Geometry check sheet. Reference: the model listing, model coordinates, mm. Round coordinates to 2 decimals unless told otherwise and drop trailing zeros. Loops run counter-clockwise (first coordinate to the right, second up) from the corner with the lowest first, then second, coordinate; pieces in that order, holes last.
```python
from build123d import *

# Parameters (mm, degrees)
F1_DEPTH = 127


with BuildPart() as f1:
    # F0 (on Top) → F1 (new body)
    with BuildSketch(Plane.XY):
        with BuildLine():
            Line((-11.57952, 10.962582), (-11.57952, 9.384583))
            ThreePointArc((-11.57952, 9.384583), (-10.88102, 9.279832), (-10.18252, 9.384583))
            Line((-10.18252, 9.384583), (-10.18252, 10.962582))
            Line((-10.18252, 10.962582), (-8.604521, 10.962582))
            ThreePointArc((-8.604521, 10.962582), (-8.49977, 11.661082), (-8.604521, 12.359582))
            Line((-8.604521, 12.359582), (-10.18252, 12.359582))
            Line((-10.18252, 12.359582), (-10.18252, 13.937582))
            ThreePointArc((-10.18252, 13.937582), (-10.88102, 14.042332), (-11.57952, 13.937582))
            Line((-11.57952, 13.937582), (-11.57952, 12.359582))
            Line((-11.57952, 12.359582), (-13.157519, 12.359582))
            ThreePointArc((-13.157519, 12.359582), (-13.26227, 11.661082), (-13.157519, 10.962582))
            Line((-13.157519, 10.962582), (-11.57952, 10.962582))
        make_face()
    extrude(amount=F1_DEPTH)


solid = f1.part
```
1) Gauge pin test, flat ends, axial feed: pin 1 (1.3 mm diameter, centred on x = -12.5, z = 59.5, fed in from -Y); pin 2 (0.8 mm diameter, centred on y = 10, z = 41.5, fed in from -X); pin 3 (0.8 mm diameter, centred on x = -12.5, z = 70.5, fed in from +Y). Record the tip position at first contact, or that the pin passes through.
Report:
pin 1: stops at y = 10.96
pin 2: stops at x = -11.58
pin 3: stops at y = 12.36
2) Sectioned sample at B-B, the plane x = -9.4. Record the cut outline in (y, z), then the cut area to 3 significant figures.
Report:
outline: (10.96, 0) - (12.36, 0) - (12.36, 127) - (10.96, 127) - close
area: 177 mm2
3) Scan lines: line 1 along X through (y, z) = (13.85, 32.5); line 2 along Y through (x, z) = (-9.05, 36.5); line 3 along X through (y, z) = (11.85, 112). Record each from-to range of solid material in increasing order.
Report:
line 1: x = -11.58 to -10.18
line 2: y = 10.96 to 12.36
line 3: x = -13.25 to -8.51
4) Sectioned sample at A-A, the plane z = 105. Record the cut outline in (x, y), then the cut area to 3 significant figures.
Report:
outline: (-13.16, 10.96) - (-11.58, 10.96) - (-11.58, 9.38) arc R2.38 ccw to (-10.18, 9.38) - (-10.18, 10.96) - (-8.6, 10.96) arc R2.38 ccw to (-8.6, 12.36) - (-10.18, 12.36) - (-10.18, 13.94) arc R2.38 ccw to (-11.58, 13.94) - (-11.58, 12.36) - (-13.16, 12.36) arc R2.38 ccw to start
area: 11.2 mm2
